```python
from build123d import *

# Parameters (mm, degrees)
BOSS_EXTRUDE1_DEPTH      = 5
BOSS_EXTRUDE1_DEPTH_BACK = 5
SKETCH1_R                = 27.5
SKETCH1_R_2              = 10
BOSS_EXTRUDE3_DEPTH      = 15
BOSS_EXTRUDE3_DEPTH_BACK = 15
SKETCH1_5_R              = 19.211681975
SKETCH1_5_R_2            = 10
SKETCH1_5_R_3            = 32
SKETCH1_5_R_4            = 27.5
BOSS_EXTRUDE4_DEPTH      = 30
BOSS_EXTRUDE4_DEPTH_BACK = 15
SKETCH1_6_R              = 21.5
SKETCH1_6_R_2            = 17
BOSS_EXTRUDE5_DEPTH      = 10
BOSS_EXTRUDE5_DEPTH_BACK = 15
SKETCH1_7_R              = 27.5
SKETCH1_7_R_2            = 21.5


with BuildPart() as part:
    # Sketch1 → Boss-Extrude1 (new, two sides: drawn at the far end of the back side and taken through both)
    with BuildSketch(Plane.XY.offset(-BOSS_EXTRUDE1_DEPTH_BACK)):
        with BuildLine():
            ThreePointArc((-26.678302647, -20.922495817), (0, -70.593606928), (26.678302647, -20.922495817))
            ThreePointArc((26.678302647, -20.922495817), (16.836772686, 4.320434327), (18.321243986, 31.373300703))
            ThreePointArc((18.321243986, 31.373300703), (0, 55.406393072), (-18.321243986, 31.373300703))
            ThreePointArc((-18.321243986, 31.373300703), (-16.836772686, 4.320434327), (-26.678302647, -20.922495817))
        make_face()
        with Locations((0, -38.593606928)):
            Circle(SKETCH1_R, mode=Mode.SUBTRACT)
        with Locations((0, 36.406393072)):
            Circle(SKETCH1_R_2, mode=Mode.SUBTRACT)
    extrude(amount=BOSS_EXTRUDE1_DEPTH + BOSS_EXTRUDE1_DEPTH_BACK)

    # Sketch1<5> → Boss-Extrude3 (add, two sides: drawn at the far end of the back side and taken through both)
    # profile 1 of 2: a face of its own
    with BuildSketch(Plane.XY.offset(-BOSS_EXTRUDE3_DEPTH_BACK)):
        with Locations((0, 36.406393072)):
            Circle(SKETCH1_5_R)
        with Locations((0, 36.406393072)):
            Circle(SKETCH1_5_R_2, mode=Mode.SUBTRACT)
    # profile 2 of 2: a face of its own
    with BuildSketch(Plane.XY.offset(-BOSS_EXTRUDE3_DEPTH_BACK)):
        with Locations((0, -38.593606928)):
            Circle(SKETCH1_5_R_3)
        with Locations((0, -38.593606928)):
            Circle(SKETCH1_5_R_4, mode=Mode.SUBTRACT)
    extrude(amount=BOSS_EXTRUDE3_DEPTH + BOSS_EXTRUDE3_DEPTH_BACK)



with BuildPart() as body_2:
    # Sketch1<6> → Boss-Extrude4 (new, two sides: drawn at the far end of the back side and taken through both)
    with BuildSketch(Plane.XY.offset(-BOSS_EXTRUDE4_DEPTH_BACK)):
        with Locations((0, -38.593606928)):
            Circle(SKETCH1_6_R)
        with Locations((0, -38.593606928)):
            Circle(SKETCH1_6_R_2, mode=Mode.SUBTRACT)
    extrude(amount=BOSS_EXTRUDE4_DEPTH + BOSS_EXTRUDE4_DEPTH_BACK)


with BuildPart() as part_1:
    add(part.part)

    add(body_2.part)  # Boss-Extrude5 merges body 2
    # Sketch1<7> → Boss-Extrude5 (add, two sides: drawn at the far end of the back side and taken through both)
    with BuildSketch(Plane.XY.offset(-BOSS_EXTRUDE5_DEPTH_BACK)):
        with Locations((0, -38.593606928)):
            Circle(SKETCH1_7_R)
        with Locations((0, -38.593606928)):
            Circle(SKETCH1_7_R_2, mode=Mode.SUBTRACT)
    extrude(amount=BOSS_EXTRUDE5_DEPTH + BOSS_EXTRUDE5_DEPTH_BACK)


solid = part_1.part
```
Build history of the part. All positions in model axes, mm. A direction names the side the tool comes from. Give positions to 0.01 mm unless a question says otherwise; leave off trailing zeros. Order: outer loops, then holes, each group sorted by start corner. A loop starts at its lowest first (then second) coordinate and runs counter-clockwise, first axis right, second up. Notation, with made-up numbers: M -0.5,43 L 21.5,43 A25 cw 21.5,60 Z; hole C -20.75,-6 d1. An arc over 180 degrees is marked long. Return JSON: item names as keys, results as strings.
Q1. Band-saw the part on C-C (z = 24). Give the cut face in (x, y).
Answer list:
{"outline": "C 0,-38.59 d43; hole C 0,-38.59 d34"}
Q2. Band-saw the part on A-A (x = 0). Give the cut face in (y, z), then the cut area to 3 significant figures.
Answer list:
{"outline": "M -70.59,-15 L -55.59,-15 L -55.59,30 L -60.09,30 L -60.09,10 L -66.09,10 L -66.09,15 L -70.59,15 Z; M -21.59,-15 L -6.59,-15 L -6.59,-5 L 17.19,-5 L 17.19,-15 L 26.41,-15 L 26.41,15 L 17.19,15 L 17.19,5 L -6.59,5 L -6.59,15 L -11.09,15 L -11.09,10 L -17.09,10 L -17.09,30 L -21.59,30 Z; M 46.41,-15 L 55.62,-15 L 55.62,15 L 46.41,15 Z", "area": "1,770 mm^2"}
Q3. 3-axis set-ups, long thin cutter, end or side, ignore diameter. For faces 1 (the face through (-2.501, 55.455, -0.21)), 2 (the face through (8, 28, -15)), 3 (the face through (-5.96, -65.44, 12.46)), 4 (the face through (8, 28, 15)), 5 (the face through (16, -32, 30)): which of +Z, -Z, +X, -X, +Y, -Y reach the whole face in a straight line?
Answer list:
{"face 1": "none", "face 2": "-Z, +X, -X, +Y, -Y", "face 3": "+Z", "face 4": "+Z, +X, -X, +Y", "face 5": "+Z, +X, -X, +Y, -Y"}
Q4. Flat gauge pins, fed straight in: pin 1 (5 mm diameter, centred on y = -46.5, z = 13, fed in from +X); pin 2 (12 mm diameter, centred on y = 33.5, z = 1.5, fed in from +X); pin 3 (5 mm diameter, centred on x = 11.5, z = -2, fed in from -Y). Where does each tip first touch, or does it go through?
Answer list:
{"pin 1": "stops at x = 31.54", "pin 2": "stops at x = 19.21", "pin 3": "stops at y = -69.3"}
Q5. Two-plate mould, pull along Y, no slides. Class faces 6 (the face through (14.1, -14.7, 15)), 7 (the face through (-1.3, 46.32, -0.21)): pulls with the +Y half, pulls with the -Y half, needs draft (parallel to the pull), parting line crosses it, or undercut.
Answer list:
{"face 6": "needs draft", "face 7": "undercut"}
Q6. Band-saw the part on B-B (y = -45.5). Give the cut face in (x, z).
Answer list:
{"outline": "M -31.25,-15 L -15.53,-15 L -15.53,30 L -20.36,30 L -20.36,10 L -26.62,10 L -26.62,15 L -31.25,15 Z; M 15.53,-15 L 31.25,-15 L 31.25,15 L 26.62,15 L 26.62,10 L 20.36,10 L 20.36,30 L 15.53,30 Z"}
Q7. Band-saw the part on D-D (y = -19). Give the cut face in (x, z).
Answer list:
{"outline": "M -25.45,-5 L -25.3,-5 L -25.3,-15 L 25.3,-15 L 25.3,-5 L 25.45,-5 L 25.45,5 L 25.3,5 L 25.3,15 L 19.3,15 L 19.3,10 L 8.85,10 L 8.85,30 L -8.85,30 L -8.85,10 L -19.3,10 L -19.3,15 L -25.3,15 L -25.3,5 L -25.45,5 Z"}
Q8. Wall check: probe 1 along Y at (x, z) = (0, 1.75); probe 2 along Y at (x, z) = (7, -4); probe 3 along Y at (x, z) = (-6, -10). Give the ranges that are in metal, low to high. Write a range as from..to.
Answer list:
{"probe 1": "y = -70.59..-55.59, -21.59..26.41, 46.41..55.62", "probe 2": "y = -69.82..-54.09, -23.1..29.26, 43.55..54.3", "probe 3": "y = -70.03..-54.5, -22.69..-7.16, 18.16..28.41, 44.41..54.66"}
